```python
from build123d import *

# Parameters (mm, degrees)
SKETCH1_R           = 10
BOSS_EXTRUDE1_DEPTH = 50
CUT_EXTRUDE6_DEPTH  = 86
CUT_EXTRUDE7_DEPTH  = 86
SKETCH4_R           = 10
CUT_EXTRUDE8_DEPTH  = 86
SKETCH5_W           = 50
SKETCH5_H           = 20
CUT_EXTRUDE9_DEPTH  = 86


with BuildPart() as part:
    # Sketch1 → Boss-Extrude1 (new body)
    with BuildSketch(Plane.XY):
        with BuildLine():
            Line((12.5, 10), (62.5, 10))
            Line((62.5, 10), (62.5, 25))
            Line((62.5, 25), (-62.5, 25))
            ThreePointArc((-62.5, 25), (-87.5, 0), (-62.5, -25))
            Line((-62.5, -25), (62.5, -25))
            Line((62.5, -25), (62.5, -10))
            Line((62.5, -10), (12.5, -10))
            Line((12.5, -10), (12.5, 10))
        make_face()
        with Locations((-62.5, 0)):
            Circle(SKETCH1_R, mode=Mode.SUBTRACT)
    extrude(amount=-BOSS_EXTRUDE1_DEPTH)

    # Sketch2 → Cut-Extrude6 (cut)
    with BuildSketch(Plane(origin=(0, 25, 0), x_dir=(1, 0, 0), z_dir=(0, 1, 0))):
        with BuildLine():
            Line((37.5, 50), (62.5, 50))
            Line((62.5, 50), (62.5, 25))
            ThreePointArc((62.5, 25), (55.17766953, 42.67766953), (37.5, 50))
        make_face()
    extrude(amount=-CUT_EXTRUDE6_DEPTH, mode=Mode.SUBTRACT)

    # Sketch3 → Cut-Extrude7 (cut)
    with BuildSketch(Plane(origin=(0, 25, 0), x_dir=(1, 0, 0), z_dir=(0, 1, 0))):
        with BuildLine():
            Line((37.5, 0), (62.5, 0))
            Line((62.5, 0), (62.5, 25))
            ThreePointArc((62.5, 25), (55.17766953, 7.32233047), (37.5, 0))
        make_face()
    extrude(amount=-CUT_EXTRUDE7_DEPTH, mode=Mode.SUBTRACT)

    # Sketch4 → Cut-Extrude8 (cut)
    with BuildSketch(Plane(origin=(0, 25, 0), x_dir=(1, 0, 0), z_dir=(0, 1, 0))):
        with Locations(Location((37.5, 25, 0), (0, 0, 270))):
            Circle(SKETCH4_R)
    extrude(amount=-CUT_EXTRUDE8_DEPTH, mode=Mode.SUBTRACT)

    # Sketch5 → Cut-Extrude9 (cut)
    with BuildSketch(Plane(origin=(0, 25, 0), x_dir=(1, 0, 0), z_dir=(0, 1, 0))):
        with Locations((-62.5, 25)):
            Rectangle(SKETCH5_W, SKETCH5_H)
    extrude(amount=-CUT_EXTRUDE9_DEPTH, mode=Mode.SUBTRACT)


solid = part.part
```
Geometry: final body of the model. Coordinates: model frame, mm. A direction names the side the tool comes from. Round coordinates to 2 decimals unless told otherwise and drop trailing zeros. Loops run counter-clockwise (first coordinate to the right, second up) from the corner with the lowest first, then second, coordinate; pieces in that order, holes last. Notation, with made-up numbers: (60, -7) -> (79, -7) arc R17 ccw to (79, 11) -> close; hole circle Ø11 at (-16.5, 86). An arc over 180 degrees is marked (long way). Write each question's results on one line, items separated by ' | '.
Item 1: Cut plane A-A on z = -5. Return the cut outline in (x, y), and give its area (3 significant figures).
Answers below:
outline: (-62.5, -25) -> (52.5, -25) -> (52.5, -10) -> (12.5, -10) -> (12.5, 10) -> (52.5, 10) -> (52.5, 25) -> (-62.5, 25) arc R25 ccw to start; hole circle Ø20 at (-62.5, 0) | area: 5,620 mm²
Item 2: Cut plane B-B on y = 0. Return the cut outline in (x, z), and give its area (3 significant figures).
Answers below:
outline: (-87.5, -50) -> (-72.5, -50) -> (-72.5, -35) -> (-87.5, -35) -> close; (-87.5, -15) -> (-72.5, -15) -> (-72.5, 0) -> (-87.5, 0) -> close; (-52.5, -50) -> (12.5, -50) -> (12.5, 0) -> (-52.5, 0) -> (-52.5, -15) -> (-37.5, -15) -> (-37.5, -35) -> (-52.5, -35) -> close | area: 3,400 mm²
Item 3: Pull-direction query (Z, two-part tool) for faces 4 (the face through (28.628, -17.395, -20.386)), 5 (the face through (-26, 0, 0)), 6 (the face through (-72.49, 0.44, -42.4)); classes: pulls with the +Z half, pulls with the -Z half, needs draft (parallel to the pull), parting line crosses it, or undercut.
Answers below:
face 4: undercut | face 5: pulls with the +Z half | face 6: needs draft
Item 4: Cut plane C-C on x = -68. Return the cut outline in (y, z), and give its area (3 significant figures).
Answers below:
outline: (-24.39, -50) -> (-8.35, -50) -> (-8.35, -35) -> (-24.39, -35) -> close; (-24.39, -15) -> (-8.35, -15) -> (-8.35, 0) -> (-24.39, 0) -> close; (8.35, -50) -> (24.39, -50) -> (24.39, -35) -> (8.35, -35) -> close; (8.35, -15) -> (24.39, -15) -> (24.39, 0) -> (8.35, 0) -> close | area: 962 mm²
Item 5: Cut plane D-D on z = -26.5. Return the cut outline in (x, y).
Answers below:
outline: (-37.5, -25) -> (27.61, -25) -> (27.61, -10) -> (12.5, -10) -> (12.5, 10) -> (27.61, 10) -> (27.61, 25) -> (-37.5, 25) -> close; (47.39, -25) -> (62.45, -25) -> (62.45, -10) -> (47.39, -10) -> close; (47.39, 10) -> (62.45, 10) -> (62.45, 25) -> (47.39, 25) -> close
Item 6: Set-up query: faces 1 (the face through (1, 25, -25)), 2 (the face through (12.5, 0, -25)), 3 (the face through (-37.5, 0, -25)). Return all of +Z, -Z, +X, -X, +Y, -Y with unobstructed straight access to the full face (end or side cutting, diameter ignored); none if empty.
Answers below:
face 1: +Z, -Z, +X, -X, +Y | face 2: +Z, -Z, +X | face 3: -X, +Y, -Y
Item 7: Line query: probe 1 along Z at (x, y) = (-53.5, -8.5); probe 2 along X at (y, z) = (-21.5, -25); probe 3 along Y at (x, z) = (-62.5, -45). Output: solid intervals per line, ascending. Write a range as [from, to].
Answers below:
probe 1: z = [-50, -35], [-15, 0] | probe 2: x = [-37.5, 27.5], [47.5, 62.5] | probe 3: y = [-25, -10], [10, 25]
Item 8: Pin query (flat end, axial travel): pin 1 Ø4 at (y, z) = (-12.5, -24) entering from -X; pin 2 Ø1.5 at (y, z) = (-16, -6) entering from +X; pin 3 Ø16 at (y, z) = (7, -27.5) entering from -X. Return the tip coordinate at first contact, or that it passes through.
Answers below:
pin 1: stops at x = -37.5 | pin 2: stops at x = 54.59 | pin 3: stops at x = -87.14
